Autodesk Inventor part; units mm, degrees
ref_plane "YZ Plane" through (0, 0, 0) normal (1, 0, 0) x (0, 1, 0)
ref_plane "XZ Plane" through (0, 0, 0) normal (0, 1, 0) x (-1, 0, 0)
ref_plane "XY Plane" through (0, 0, 0) normal (0, 0, 1) x (1, 0, 0)
ref_plane "작업 평면1" through (0, 0, 0) normal (0, 0, 1) x (1, 0, 0)
sketch "스케치1" plane through (0, 0, 0) normal (0, 0, 1) x (1, 0, 0)
  line L0 (6.3, 9.65) -> (6.3, 14.85)
  line L1 (4.1, 9.65) -> (6.3, 9.65)
  line L2 (4.1, 14.85) -> (4.1, 9.65)
  line L3 (6.3, 14.85) -> (4.1, 14.85)
  line L4 (4.1, -7.15) -> (4.1, -12.35)
  line L5 (6.3, -7.15) -> (4.1, -7.15)
  line L6 (6.3, -12.35) -> (6.3, -7.15)
  line L7 (4.1, -12.35) -> (6.3, -12.35)
  line L8 (10.2, -17.75) -> (-10.2, -17.75)
  line L9 (10.2, 17.75) -> (10.2, -17.75)
  line L10 (-10.2, 17.75) -> (10.2, 17.75)
  line L11 (-10.2, -17.75) -> (-10.2, 17.75)
  circle A0 centre (-7.5, 14.75) radius 1.35
  circle A1 centre (-7.5, -7.25) radius 1.35
  line L12 (-10.2, 17.75) -> (10.2, 17.75)
  line L13 (10.2, 17.75) -> (10.2, -17.75)
  line L14 (10.2, -17.75) -> (-10.2, -17.75)
  line L15 (-10.2, -17.75) -> (-10.2, 17.75)
  point P0 (0, 0)
extrude "돌출1" add sketch "스케치1" against normal blind 3
ref_plane "작업 평면2" through (10.2, 17.75, -3) normal (1, 0, 0) x (0, -1, 0)
sketch "스케치2" plane through (10.2, 17.75, -3) normal (1, 0, 0) x (0, -1, 0)
  circle A0 centre (27.5, -0.3) radius 1.35
  circle A1 centre (5.5, -0.3) radius 1.35
  line L0 (35.5, 2.4) -> (35.5, -3)
  line L1 (0, 2.4) -> (35.5, 2.4)
  line L2 (0, 2.4) -> (0, -3)
  line L3 (0, -3) -> (35.5, -3)
  line L4 (0, -3) -> (35.5, -3)
  line L5 (35.5, -3) -> (35.5, 2.4)
  line L6 (35.5, 2.4) -> (0, 2.4)
  line L7 (0, 2.4) -> (0, -3)
  point P0 (17.75, -3)
extrude "돌출2" add sketch "스케치2" against normal blind 12
sketch "스케치3" plane through (10.2, -17.75, 0) normal (1, 0, 0) x (0, 0, -1)
  circle A0 centre (2.7, 8) radius 1.35
  circle A1 centre (2.7, 30) radius 1.35
  line L0 (5.4, 0) -> (0, 0)
  line L1 (5.4, 35.5) -> (5.4, 0)
  line L2 (5.4, 35.5) -> (0, 35.5)
  line L3 (0, 35.5) -> (0, 0)
  circle A2 centre (2.7, 30) radius 1.35
  circle A3 centre (2.7, 8) radius 1.35
  point P0 (0, 17.75)
extrude "돌출3" cut sketch "스케치3" against normal blind 12 contours A0 | A1
properties part number "dehind ankle connection_inside" material "PMMA 플라스틱"
Design review of the part built by this model. Coordinates are the model's own, in mm. A direction names the side the tool comes from. Give positions to 0.01 mm unless a question says otherwise; leave off trailing zeros. Order: outer loops, then holes, each group sorted by start corner. A loop starts at its lowest first (then second) coordinate and runs counter-clockwise, first axis right, second up. Notation, with made-up numbers: (36, 31.5) - (59, 31.5) arc R20 cw to (59, 37.5) - close; hole circle Ø8 at (-21, -1). An arc over 180 degrees is marked (long way). Use CSV: the item, a comma, the result in double quotes. Start each with the question number.
Q1. Machinability: for faces 1 (the face through (2, -17.75, -2)), 2 (the face through (-1.8, 0, -4)), 3 (the face through (4.284, 10.923, -2.454)), which of the approach directions +Z, -Z, +X, -X, +Y, -Y give a long, thin tool a straight path to every point of the face, cutting with its end or side? Answer none if there is none.
Q2. For line 1 (Y direction, x = -7.5, z = -1); line 2 (Y direction, x = 5, z = -2.7); line 3 (Z direction, x = -9, y = -4), list the stretches that pass through material, from the lowest coordinate up.
Q3. Take a section at B-B (z = -3.6). State the section outline as (x, y) points, and give its area (3 significant figures).
Q4. Take a section at D-D (x = 2). State the section outline as (y, z) points.
Q5. Take a section at C-C (y = 9.5). State the section outline as (x, z) points, and give its area (3 significant figures).
Q6. For P1, Ø2.5, axis at y = -6.5, z = -4.5, coming from the -X side; P2, Ø6.5, axis at x = -5.5, y = -8.5, coming from the -Z side; P3, Ø0.5, axis at y = 13, z = -2, coming from the +X side, all flat-tipped, find the tip position at first contact; note any pin that passes through.
Q7. Take a section at A-A (y = 14.75). State the section outline as (x, z) points, and give its area (3 significant figures).
Q8. Draft analysis for pull direction Z (two halves, no side actions). For faces 4 (the face through (10.2, 0, -3)), 5 (the face through (-1.8, 12, -2)), 6 (the face through (4, 0, -5.4)), state which applies: pulls with the +Z half, pulls with the -Z half, needs draft (parallel to the pull), parting line crosses it, or undercut.
Calculated:
1,face 1,"+Z, -Z, +X, -X, -Y"
1,face 2,"-Z, -X, +Y, -Y"
1,face 3,"+X"
2,line 1,"y = -17.75 to -8.6, -5.9 to 13.4, 16.1 to 17.75"
2,line 2,"y = -17.75 to -11.1, -8.4 to 10.9, 13.6 to 17.75"
2,line 3,"z = -3 to 0"
3,outline,"(-1.8, -17.75) - (10.2, -17.75) - (10.2, -10.76) - (-1.8, -10.76) - close; (-1.8, -8.74) - (10.2, -8.74) - (10.2, 11.24) - (-1.8, 11.24) - close; (-1.8, 13.26) - (10.2, 13.26) - (10.2, 17.75) - (-1.8, 17.75) - close"
3,area,"378 mm²"
4,outline,"(-17.75, -5.4) - (17.75, -5.4) - (17.75, 0) - (-17.75, 0) - close; hole circle Ø2.7 at (-9.75, -2.7); hole circle Ø2.7 at (12.25, -2.7)"
5,outline,"(-10.2, -3) - (-1.8, -3) - (-1.8, -5.4) - (10.2, -5.4) - (10.2, 0) - (-10.2, 0) - close"
5,area,"90.0 mm²"
6,P1,"stops at x = -1.8"
6,P2,"stops at z = -3"
6,P3,"stops at x = -1.8"
7,outline,"(-10.2, -3) - (-8.85, -3) - (-8.85, 0) - (-10.2, 0) - close; (-6.15, -3) - (-1.8, -3) - (-1.8, -5.4) - (10.2, -5.4) - (10.2, 0) - (-6.15, 0) - close"
7,area,"81.9 mm²"
8,face 4,"needs draft"
8,face 5,"undercut"
8,face 6,"pulls with the -Z half"
